from build123d import *

# Parameters (mm, degrees)
F0_R     = 38.1
F0_R_2   = 12.7
F1_DEPTH = 15
F2_SIZE  = 2
F5_D     = 8.8
F5_DEPTH = 38.1
F5_TIP   = 2.6437867237


# Not quite as in the source:
# - a length typed as a fraction of an inch, garbled in the dataset ("3 / 203.2 mm" for 3/8 in), is restored


with BuildPart() as f1:
    # F0 (on Top) → F1 (new body)
    with BuildSketch(Plane.XY):
        Circle(F0_R)
        Circle(F0_R_2, mode=Mode.SUBTRACT)
    extrude(amount=F1_DEPTH)

    # F2
    f2_edges = [f1.edges().sort_by_distance(p)[0] for p in [
        (-38.1, 0, 15),
        (-38.1, 0, 0),
    ]]
    chamfer(f2_edges, length=F2_SIZE)

    # F5
    with Locations(Plane.YZ.offset(38.1)):
        with Locations((0, 7.5)):
            Hole(F5_D / 2, depth=F5_DEPTH)
            with Locations((0, 0, -(F5_DEPTH + F5_TIP / 2))):  # 118° drill point
                Cone(0, F5_D / 2, F5_TIP, mode=Mode.SUBTRACT)


solid = f1.part
Verification items for the finished model (mm, model axes). Coordinates: 2 decimals unless noted, no trailing zeros. Write each loop counter-clockwise with the first axis right and the second up, starting at its lowest first coordinate (ties: lowest second). Pieces come first, ordered by that corner, then holes. Notation, with made-up numbers: M -20.5,-25.75 L 30.5,-25.75 A21 ccw 30.5,-11.75 Z; hole C -23,6 d3. An arc over 180 degrees is marked long. Use a Markdown table: item, result.
Q1. Thickness scan on line 1 (Y direction, x = 0, z = 10.75); line 2 (X direction, y = 4.5, z = 0.75); line 3 (Y direction, x = 18.75, z = 7.5). Record the ranges inside material, lowest first.
Reply:
| item | result |
|---|---|
| line 1 | y = -38.1 to -12.7, 12.7 to 38.1 |
| line 2 | x = -36.57 to -11.88, 11.88 to 36.57 |
| line 3 | y = -33.17 to -4.4, 4.4 to 33.17 |
Q2. Sectioned sample at C-C, the plane z = 7.5. Record the boundary of the cut face in (x, y), plus the area to 3 significant figures.
Reply:
| item | result |
|---|---|
| outline | M 11.91,-4.4 A12.7 cw long 11.91,4.4 L 37.85,4.4 A38.1 ccw long 37.85,-4.4 Z |
| area | 3,830 mm² |
Q3. Sectioned sample at B-B, the plane y = 0. Record the boundary of the cut face in (x, z).
Reply:
| item | result |
|---|---|
| outline | M -38.1,2 L -36.1,0 L -12.7,0 L -12.7,15 L -36.1,15 L -38.1,13 Z; M 12.7,0 L 36.1,0 L 38.1,2 L 38.1,3.1 L 12.7,3.1 Z; M 12.7,11.9 L 38.1,11.9 L 38.1,13 L 36.1,15 L 12.7,15 Z |
Q4. Sectioned sample at A-A, the plane x = 0. Record the boundary of the cut face in (y, z), plus the area to 3 significant figures.
Reply:
| item | result |
|---|---|
| outline | M -38.1,2 L -36.1,0 L -12.7,0 L -12.7,15 L -36.1,15 L -38.1,13 Z; M 12.7,0 L 36.1,0 L 38.1,2 L 38.1,13 L 36.1,15 L 12.7,15 Z |
| area | 754 mm² |
Q5. Draft check along Y on faces 1 (the face through (-30.235, -23.183, 7.423)), 2 (the face through (-10.1, -7.7, 7.4)), 3 (the face through (-1, -16, 0)), 4 (the face through (24.823, 0.954, 3.205)). Enter one of: +Y half, -Y half, draft (parallel to the pull), parting line (faces both ways), or undercut.
Reply:
| item | result |
|---|---|
| face 1 | parting line |
| face 2 | undercut |
| face 3 | draft |
| face 4 | undercut |
Q6. Go/stop test with flat-tipped pins: P1, Ø3, axis at y = 18, z = 13, coming from the -X side; P2, Ø4, axis at x = -18, z = 11.5, coming from the -Y side; P3, Ø8, axis at x = -19, z = 5, coming from the +Y side. Record where each tip stops, or that it passes through.
Reply:
| item | result |
|---|---|
| P1 | stops at x = -34.34 |
| P2 | stops at y = -34.58 |
| P3 | stops at y = 35.02 |
